The figure shows three views and two pictorial views of one solid part (mm, origin at its lowest corner). Answer the questions. Give positions to 0.01 mm unless a question says otherwise; leave off trailing zeros. Order: outer loops, then holes, each group sorted by start corner. A loop starts at its lowest first (then second) coordinate and runs counter-clockwise, first axis right, second up. Notation, with made-up numbers: (-29, -8.5) -> (-21, -8.5) arc R22 ccw to (-21, 18.5) -> close; hole circle Ø9 at (-20.75, -6). An arc over 180 degrees is marked (long way). Use one line per item in the form item = value.
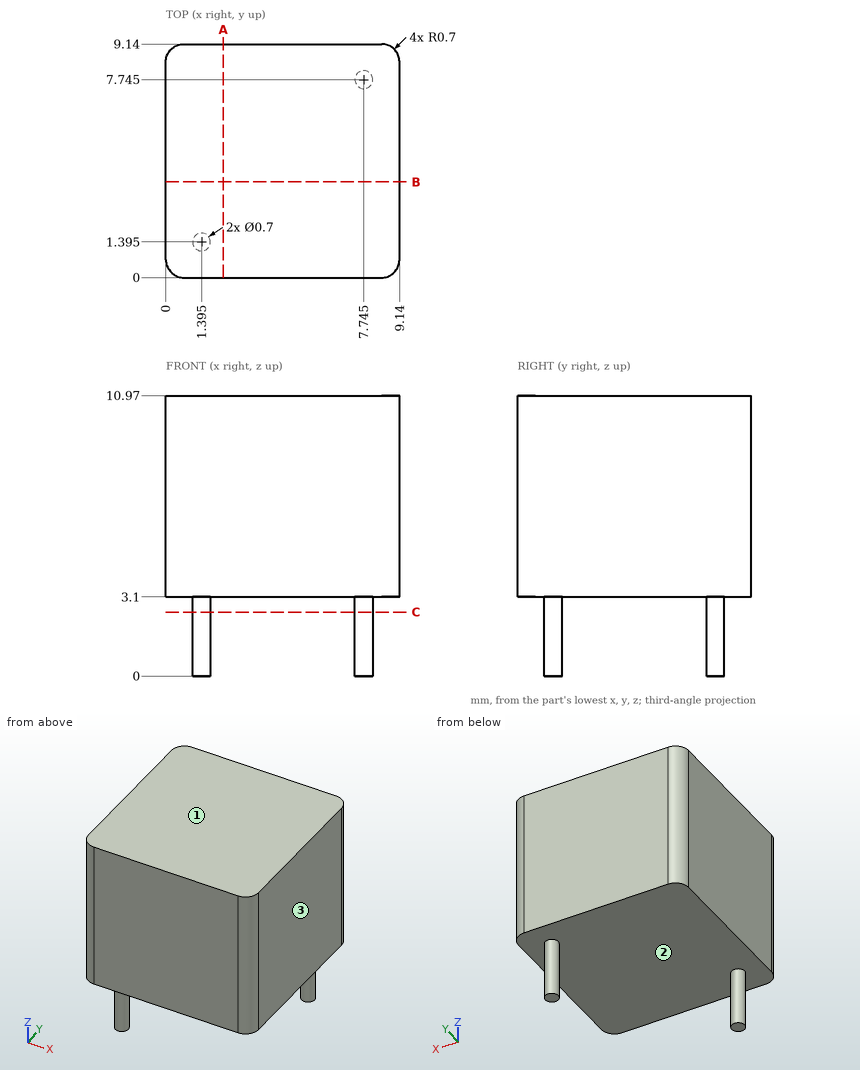
Item 1: Determine the mould class of the marked faces 1, 2 and 3 for opening direction Z: +Z half, -Z half, draft (parallel to the pull), parting line (faces both ways), or undercut.
Checks:
face_1 = +Z half
face_2 = -Z half
face_3 = draft
Item 2: The part is cut by section C-C on z = 2.5. Give the vertices of the cut face in (x, y) (3 decimals), and give its area (3 significant figures).
Checks:
outline = circle Ø0.7 at (1.395, 1.395); circle Ø0.7 at (7.745, 7.745)
area = 0.770 mm²
Item 3: Given pin 1 Ø4 at (x, z) = (6, 2.5) entering from -Y; pin 2 Ø4.5 at (x, y) = (3, 3.5) entering from -Z, each flat-ended and moving along its own axis, determine where each tip first touches the part or whether it passes through.
Checks:
pin_1 = 0
pin_2 = 3.1
Item 4: The part is cut by section A-A on x = 2.25. Give the vertices of the cut face in (y, z), and give its area (3 significant figures).
Checks:
outline = (0, 3.1) -> (9.14, 3.1) -> (9.14, 10.97) -> (0, 10.97) -> close
area = 71.9 mm²
Item 5: Straight lines are drawn through the part: L1, parallel to Z at x = 0.5, y = 4.75; L2, parallel to X at y = 7.5, z = 1. For each, find the intervals that lie inside material, in ascending order. Write a range as from..to.
Checks:
L1 = 3.1..10.97
L2 = 7.5..7.99
